CAD build for the part. Positions are in the model's coordinates, mm. A direction names the side the tool comes from. Coordinates: 2 decimals unless noted, no trailing zeros. Order: outer loops, then holes, each group sorted by start corner. A loop starts at its lowest first (then second) coordinate and runs counter-clockwise, first axis right, second up. Notation, with made-up numbers: M 72,59 L 123,59 A17 ccw 123,65 Z; hole C -11.75,31 d6. An arc over 180 degrees is marked long. Write item = value, one per line.
from build123d import *

# Parameters (mm, degrees)
SKETCH1_R                      = 12.5
BOSS_EXTRUDE1_DEPTH            = 17.6
SKETCH2_R                      = 6.875
CUT_EXTRUDE1_DEPTH             = 50.8
SKETCH3_R                      = 8.875
CUT_EXTRUDE3_DEPTH             = 15.6
CUT_EXTRUDE4_DEPTH             = 18.6
BOSS_EXTRUDE2_DEPTH            = 17.6
FILLET1_R                      = 4
SKETCH6_W                      = 25
SKETCH6_H                      = 20.775
BOSS_EXTRUDE3_DEPTH            = 20
M4X0_7_TAPPED_HOLE2_AT_2_COUNT = 2
M4X0_7_TAPPED_HOLE2_AT_2_PITCH = 12.206555616
M4X0_7_TAPPED_HOLE1_D          = 3.3
M4X0_7_TAPPED_HOLE1_DEPTH      = 7
M4X0_7_TAPPED_HOLE1_TIP        = 0.991420021
FILLET4_R                      = 1
FILLET6_R                      = 1
FILLET7_R                      = 2
CUT_EXTRUDE6_DEPTH             = 15.6
FILLET8_R                      = 5
BOSS_EXTRUDE4_DEPTH            = 17.6
CUT_EXTRUDE8_DEPTH             = 18.6000001
CUT_EXTRUDE9_DEPTH             = 18.6000001
CUT_EXTRUDE10_DEPTH            = 15.6
FILLET10_R                     = 1
FILLET12_R                     = 1
FILLET13_R                     = 2


with BuildPart() as part:
    # Sketch1 → Boss-Extrude1 (new body)
    with BuildSketch(Plane(origin=(0, 0, 0), x_dir=(1, 0, 0), z_dir=(0, 1, 0))):
        Circle(SKETCH1_R)
    extrude(amount=BOSS_EXTRUDE1_DEPTH)

    # Sketch2 → Cut-Extrude1 (cut)
    with BuildSketch(Plane(origin=(0, 17.6, 0), x_dir=(1, 0, 0), z_dir=(0, 1, 0))):
        Circle(SKETCH2_R)
    extrude(amount=-CUT_EXTRUDE1_DEPTH, mode=Mode.SUBTRACT)

    # Sketch3 → Cut-Extrude3 (cut)
    with BuildSketch(Plane(origin=(0, 17.6, 0), x_dir=(1, 0, 0), z_dir=(0, 1, 0))):
        Circle(SKETCH3_R)
    extrude(amount=-CUT_EXTRUDE3_DEPTH, mode=Mode.SUBTRACT)

    # Sketch4 → Cut-Extrude4 (cut, through all)
    with BuildSketch(Plane(origin=(0, 17.6, 0), x_dir=(1, 0, 0), z_dir=(0, 1, 0))):
        with BuildLine():
            ThreePointArc((-3.035428772, 8.339772009), (2.668763971, 8.464237938), (7.269974393, 5.090490873))
            Line((7.269974393, 5.090490873), (10.239400554, 7.169705454))
            ThreePointArc((10.239400554, 7.169705454), (3.758822494, 11.921461884), (-4.275251792, 11.74615776))
            Line((-4.275251792, 11.74615776), (-3.035428772, 8.339772009))
        make_face()
    extrude(amount=-CUT_EXTRUDE4_DEPTH, mode=Mode.SUBTRACT)

    # Sketch5 → Boss-Extrude2 (add, through all)
    with BuildSketch(Plane(origin=(0, 17.6, 0), x_dir=(1, 0, 0), z_dir=(0, 1, 0))):
        with BuildLine():
            Line((8.100371818, -9.520187835), (32.472052675, 11.216764019))
            Line((32.472052675, 11.216764019), (23.399636239, 21.879374394))
            Line((23.399636239, 21.879374394), (10.717665156, 11.088759446))
            Line((10.717665156, 11.088759446), (10.239400554, 7.169705454))
            ThreePointArc((10.239400554, 7.169705454), (12.398586499, -1.589041484), (8.100371818, -9.520187835))
        make_face()
    extrude(amount=-BOSS_EXTRUDE2_DEPTH)

    # Fillet1
    fillet1_edges = [part.edges().sort_by_distance(p)[0] for p in [
        (-3.035428772, 9.8, -8.339772009),
    ]]
    fillet(fillet1_edges, radius=FILLET1_R)

    # Sketch6 → Boss-Extrude3 (add)
    with BuildSketch(Plane(origin=(24.371680857, 0, -20.736951854), x_dir=(-0.648029745, 0, -0.761615027), z_dir=(0.761615027, 0, -0.648029745))):
        with Locations((0, 10.3875)):
            Rectangle(SKETCH6_W, SKETCH6_H)
    extrude(amount=BOSS_EXTRUDE3_DEPTH)

    # Sketch9 → M4x0.7 Tapped Hole2 (revolve, cut)
    with BuildSketch(Plane(origin=(25.410689361, 15.3875, -38.033496634), x_dir=(-0.761615027, 0, 0.648029745), z_dir=(0, 1, 0))):
        Polygon((0, 0), (0, 7.991420021), (1.65, 7), (1.65, 0), align=None)
    m4x0_7_tapped_hole2 = revolve(axis=Axis((21.295700477, 15.3875, -42.869752054), (0.648029745, 0, 0.761615027)), mode=Mode.SUBTRACT)

    # M4x0.7 Tapped Hole2 at 2: M4x0.7 Tapped Hole2 ×2
    with Locations(*[Vector(-0.436757539, -0.819231921, 0.371620657) * (i * M4X0_7_TAPPED_HOLE2_AT_2_PITCH) for i in range(1, M4X0_7_TAPPED_HOLE2_AT_2_COUNT)]):
        add(m4x0_7_tapped_hole2, mode=Mode.SUBTRACT)

    # Mirror1: M4x0.7 Tapped Hole2 across plane
    add(m4x0_7_tapped_hole2.mirror(Plane(origin=(0, 0, 0), x_dir=(-0.761615027, 0, 0.648029745), z_dir=(-0.648029745, 0, -0.761615027))), mode=Mode.SUBTRACT)

    # Mirror1 copy 1 sketch → Mirror1 copy 1 (revolve, cut)
    with BuildSketch(Plane(origin=(36.280127809, 5.3875, -14.456912746), x_dir=(-0.761615027, 0, 0.648029745), z_dir=(0, 1, 0))):
        Polygon((0, 0), (0, -7.991420021), (1.65, -7), (1.65, 0), align=None)
    revolve(axis=Axis((40.395116693, 5.3875, -9.620657326), (0.648029745, 0, 0.761615027)), mode=Mode.SUBTRACT)

    # M4x0.7 Tapped Hole1
    with Locations(Plane(origin=(0, 17.6, 0), x_dir=(1, 0, 0), z_dir=(0, 1, 0))):
        with Locations((20.785019884, 12.607162838), (15.760988598, 3.080405276)):
            Hole(M4X0_7_TAPPED_HOLE1_D / 2, depth=M4X0_7_TAPPED_HOLE1_DEPTH)
            with Locations((0, 0, -(M4X0_7_TAPPED_HOLE1_DEPTH + M4X0_7_TAPPED_HOLE1_TIP / 2))):  # 118° drill point
                Cone(0, M4X0_7_TAPPED_HOLE1_D / 2, M4X0_7_TAPPED_HOLE1_TIP, mode=Mode.SUBTRACT)

    # Fillet4
    fillet4_edges = [part.edges().sort_by_distance(p)[0] for p in [
        (27.935844457, 17.6, -16.548069207),
    ]]
    fillet(fillet4_edges, radius=FILLET4_R)

    # Fillet6
    fillet6_edges = [part.edges().sort_by_distance(p)[0] for p in [
        (-3.035428772, 1, -8.339772009),
        (7.269974393, 1, -5.090490873),
    ]]
    fillet(fillet6_edges, radius=FILLET6_R)

    # Fillet7
    fillet7_edges = [part.edges().sort_by_distance(p)[0] for p in [
        (23.399636239, 8.8, -21.879374394),
    ]]
    fillet(fillet7_edges, radius=FILLET7_R)

    # Sketch13 → Cut-Extrude6 (cut)
    with BuildSketch(Plane(origin=(0, 17.6, 0), x_dir=(1, 0, 0), z_dir=(0, 1, 0))):
        Polygon((8.029469851, 3.780640013), (11.336580589, 16.160351586), (5.704740036, 6.798644433), (7.043250731, 5.399837418), align=None)
    extrude(amount=-CUT_EXTRUDE6_DEPTH, mode=Mode.SUBTRACT)

    # Fillet8
    fillet8_edges = [part.edges().sort_by_distance(p)[0] for p in [
        (8.029469851, 9.8, -3.780640013),
    ]]
    fillet(fillet8_edges, radius=FILLET8_R)

    # Sketch14 → Boss-Extrude4 (add)
    with BuildSketch(Plane(origin=(0, 17.6, 0), x_dir=(1, 0, 0), z_dir=(0, 1, 0))):
        Polygon((8.634649617, 6.046046752), (9.642801422, 9.819923576), (10.717665156, 11.088759446), (10.239400554, 7.169705454), align=None)
    extrude(amount=-BOSS_EXTRUDE4_DEPTH)

    # Sketch15 → Cut-Extrude8 (cut, through all)
    with BuildSketch(Plane(origin=(0, 17.6, 0), x_dir=(1, 0, 0), z_dir=(0, 1, 0))):
        with BuildLine():
            Line((8.100371818, -9.520187835), (11.149703632, -6.925625425))
            Line((11.149703632, -6.925625425), (8.182097481, -3.437863553))
            ThreePointArc((8.182097481, -3.437863553), (-6.728578701, -5.787214672), (-2.175290984, 8.6042858))
            Line((-2.175290984, 8.6042858), (-4.275251792, 11.74615776))
            ThreePointArc((-4.275251792, 11.74615776), (-10.803807178, -6.287109865), (8.100371818, -9.520187835))
        make_face()
    extrude(amount=-CUT_EXTRUDE8_DEPTH, mode=Mode.SUBTRACT)

    # Sketch16 → Cut-Extrude9 (cut, through all)
    with BuildSketch(Plane(origin=(0, 17.6, 0), x_dir=(1, 0, 0), z_dir=(0, 1, 0))):
        Polygon((8.182097481, -3.437863553), (11.149703632, -6.925625425), (14.637465505, -3.958019274), align=None)
    extrude(amount=-CUT_EXTRUDE9_DEPTH, mode=Mode.SUBTRACT)

    # Sketch17 → Cut-Extrude10 (cut)
    with BuildSketch(Plane(origin=(0, 17.6, 0), x_dir=(1, 0, 0), z_dir=(0, 1, 0))):
        Polygon((8.738215958, 6.433733022), (10.661432187, -3.637641494), (8.182097481, -3.437863553), (7.951366346, 5.910414581), align=None)
    extrude(amount=-CUT_EXTRUDE10_DEPTH, mode=Mode.SUBTRACT)

    # Fillet10
    fillet10_edges = [part.edges().sort_by_distance(p)[0] for p in [
        (8.634649617, 1, -6.046046752),
    ]]
    fillet(fillet10_edges, radius=FILLET10_R)

    # Fillet12
    fillet12_edges = [part.edges().sort_by_distance(p)[0] for p in [
        (9.699824072, 2, -1.398045764),
    ]]
    fillet(fillet12_edges, radius=FILLET12_R)

    # Fillet13
    fillet13_edges = [part.edges().sort_by_distance(p)[0] for p in [
        (8.182097481, 1, 3.437863553),
        (14.637465505, 8.8, 3.958019274),
    ]]
    fillet(fillet13_edges, radius=FILLET13_R)


solid = part.part
(1) Slice it at A-A, the plane x = 0. Write the cut outline in (y, z) (3 decimals).
Evaluation:
outline = M 0,-8.875 L 2,-8.875 L 2,-6.875 L 0,-6.875 Z; M 0,6.875 L 2,6.875 L 2,8.875 L 0,8.875 Z
(2) Pin check, flat tips, straight feed: pin 1 Ø2 at (y, z) = (17.5, -25) entering from +X; pin 2 Ø4 at (y, z) = (10.5, -30) entering from +X; pin 3 Ø5.5 at (x, z) = (15.76, -3.08) entering from +Y; pin 4 Ø8 at (x, y) = (6, 17.5) entering from -Z. Stop position of each tip, or through.
Evaluation:
pin_1 = 47.7
pin_2 = 44.45
pin_3 = 17.6
pin_4 = -10.24
(3) Wall check: line 1 (Z direction, x = 0, y = 0.7) (3 decimals); line 2 (X direction, y = 0.45, z = 0) (3 decimals); line 3 (X direction, y = 11, z = -4.5). Give the ranges that are in metal, low to high. Write a range as from..to.
Evaluation:
line_1 = -8.875..-6.875, 6.875..8.875
line_2 = -8.875..-6.875, 6.875..19.289
line_3 = 9.11..14.92, 16.6..24.58
(4) Pull direction Y, two halves, no side cores. Call faces 6 (the face through (16.375, 8.923, -15.902)), 7 (the face through (27, 17.9, -17.21)), 8 (the face through (39.6, 17, -21.9)): +Y half, -Y half, draft (parallel to the pull), parting line (faces both ways), or undercut.
Evaluation:
face_6 = draft
face_7 = +Y half
face_8 = undercut
(5) Slice it at B-B, the plane y = 12.25. Write the cut outline in (x, z), then the cut area to 3 significant figures.
Evaluation:
outline = M 8.74,-6.43 L 9.64,-9.82 L 10.72,-11.09 L 21.88,-20.58 A2 cw 22.1,-23.4 L 16.27,-30.26 L 31.5,-43.22 L 47.7,-24.18 L 15.27,3.42 A2 ccw 13.81,3.89 L 10.66,3.64 Z; hole C 15.76,-3.08 d3.3; hole C 20.79,-12.61 d3.3
area = 809 mm²
(6) Tool access for faces 1 (the face through (20.885, 12.841, -24.835)), 2 (the face through (18, 17.6, -9)), 3 (the face through (31, 5, -20)), 4 (the face through (12.17, 8.92, 3.76)), 5 (the face through (19.26, 14.05, -11.98)): list every direction of +Z, -Z, +X, -X, +Y, -Y with a clear straight run to the whole face (end or side of a thin tool).
Evaluation:
face_1 = -X, +Y
face_2 = +Z, -X, +Y
face_3 = none
face_4 = +Z, +Y, -Y
face_5 = +Y
